The model under review builds one solid part; all positions refer to its coordinate system, in mm. A direction names the side the tool comes from. Give positions to 0.01 mm unless a question says otherwise; leave off trailing zeros. Order: outer loops, then holes, each group sorted by start corner. A loop starts at its lowest first (then second) coordinate and runs counter-clockwise, first axis right, second up. Notation, with made-up numbers: (30, 53.25) - (67, 53.25) arc R8 ccw to (67, 66.25) - close; hole circle Ø5 at (-4.5, 22). An arc over 180 degrees is marked (long way). Write item = value, one per line. Start each with the question number.
1. Machinability: for faces 5 (the cylindrical face through (2.93, 2.12, 10.96)), 6 (the flat face through (-7, -6.9, 6)), 7 (the cylindrical face through (-0.709, 5.828, 3.636)), 8 (the flat face through (16.675, -2, 6)), which of the approach directions +Z, -Z, +X, -X, +Y, -Y give a long, thin tool a straight path to every point of the face, cutting with its end or side? Answer none if there is none.
2. We need section C-C, the plane z = 2.25. Give the boundary of the cut face in (x, y) (3 decimals), and give its area (3 significant figures).
3. We need section B-B, the plane x = -8.5. Give the boundary of the cut face in (y, z).
4. Wall thickness on probe 1 along Y at (x, z) = (-5, 4); probe 2 along X at (y, z) = (-15, 3.5) (3 decimals); probe 3 along Y at (x, z) = (12.5, 1): over which ranges is each line inside the solid? List them lowest first.
5. We need section D-D, the plane x = 7. Give the boundary of the cut face in (y, z), and give its area (3 significant figures).
6. Mouldability with a two-part tool opening along X and no side actions: class faces 1 (the cylindrical face through (-7.226, -5.632, 5.994)), 2 (the flat face through (-10.925, -6, 9)), 3 (the flat face through (5, -12, 0)), 4 (the cylindrical face through (17.776, -5.632, 5.994)) as pulls with the +X half, pulls with the -X half, needs draft (parallel to the pull), parting line crosses it, or undercut.
7. We need section A-A, the plane y = 1. Give the boundary of the cut face in (x, z) (3 decimals), and give its area (3 significant figures).
8. For P1, Ø5, axis at x = 17.5, z = 10.5, coming from the +Y side; P2, Ø4, axis at x = -9.5, z = 4, coming from the -Y side; P3, Ø4, axis at y = -17, z = 2, coming from the -X side (3 decimals), all flat-tipped, find the tip position at first contact; note any pin that passes through.
from build123d import *

# Parameters (mm, degrees)
BOSS_EXTRUDE1_DEPTH = 11.85
BOSS_EXTRUDE2_DEPTH = 4.3
SKETCH4_R           = 2.35
BOSS_EXTRUDE3_DEPTH = 31.3
CUT_EXTRUDE1_DEPTH  = 32.1


with BuildPart() as part:
    # Sketch1 → Boss-Extrude1 (new body)
    with BuildSketch(Plane.XY):
        Polygon((0, 0), (-6.125, 0), (-6.125, -4.4), (-10.925, -4.4), (-10.925, -6.9), (-6.125, -6.9), (-6.125, -23.9), (16.675, -23.9), (16.675, -6.9), (21.175, -6.9), (21.175, -4.4), (16.675, -4.4), (16.675, 0), align=None)
    extrude(amount=BOSS_EXTRUDE1_DEPTH)

    # Boss-Extrude2: read off the stored shape, not the designer's step
    # Boss-Extrude2 outline → Boss-Extrude2 (add)
    with BuildSketch(Plane(origin=(0, 0, 0), x_dir=(1, 0, 0), z_dir=(0, 1, 0))):
        with BuildLine():
            Line((5.048154438, -8.68), (5.62, -8.68))
            ThreePointArc((5.62, -8.68), (8.37, -5.93), (5.62, -3.18))
            Line((5.62, -3.18), (5.048154438, -3.18))
            ThreePointArc((5.048154438, -3.18), (-5.20541828, -2.759603678), (-0.44336187, -11.85))
            Line((-0.44336187, -11.85), (0.04336187, -11.85))
            ThreePointArc((0.04336187, -11.85), (2.970396322, -10.93541828), (5.048154438, -8.68))
        make_face()
    extrude(amount=BOSS_EXTRUDE2_DEPTH)

    # Sketch4 → Boss-Extrude3 (add)
    with BuildSketch(Plane.XZ.offset(23.9)):
        with Locations((-0.2, 5.93)):
            Circle(SKETCH4_R)
    extrude(amount=-BOSS_EXTRUDE3_DEPTH)

    # Sketch5 → Cut-Extrude1 (cut)
    with BuildSketch(Plane(origin=(0, -4.4, 0), x_dir=(1, 0, 0), z_dir=(0, 1, 0))):
        with BuildLine():
            Line((-10.137435839, -5.425), (-10.925, -5.425))
            Line((-10.925, -5.425), (-10.925, -5.925))
            Line((-10.925, -5.925), (-10.925, -6.425))
            Line((-10.925, -6.425), (-10.140971398, -6.425))
            ThreePointArc((-10.140971398, -6.425), (-7.225009375, -5.935303305), (-10.137435839, -5.425))
        make_face()
        with BuildLine():
            Line((20.687435839, -5.425), (21.475, -5.425))
            Line((21.475, -5.425), (21.475, -5.925))
            Line((21.475, -5.925), (21.475, -6.425))
            Line((21.475, -6.425), (20.690971398, -6.425))
            ThreePointArc((20.690971398, -6.425), (17.775009375, -5.935303305), (20.687435839, -5.425))
        make_face()
    extrude(amount=-CUT_EXTRUDE1_DEPTH, mode=Mode.SUBTRACT)


solid = part.part
Model answer:
q1.face_5 = +Z, +X, +Y
q1.face_6 = +Z, -Z, -X, -Y
q1.face_7 = +Y
q1.face_8 = +Z, -Z, +X, +Y
q2.outline = (-10.925, -6.9) - (-6.125, -6.9) - (-6.125, -23.9) - (16.675, -23.9) - (16.675, -6.9) - (21.175, -6.9) - (21.175, -4.4) - (16.675, -4.4) - (16.675, 0) - (4.444, 0) - (4.444, 4.3) - (-4.844, 4.3) - (-4.844, 0) - (-6.125, 0) - (-6.125, -4.4) - (-10.925, -4.4) - close
q2.area = 608 mm2
q3.outline = (-6.9, 0) - (-4.4, 0) - (-4.4, 4.45) - (-6.9, 4.45) - close; (-6.9, 7.41) - (-4.4, 7.41) - (-4.4, 11.85) - (-6.9, 11.85) - close
q4.probe_1 = -23.9 to 4.3
q4.probe_2 = -6.125 to 16.675
q4.probe_3 = -23.9 to 0
q5.outline = (-23.9, 0) - (0, 0) - (0, 3.55) - (4.3, 3.55) - (4.3, 8.31) - (0, 8.31) - (0, 11.85) - (-23.9, 11.85) - close
q5.area = 304 mm2
q6.face_1 = undercut
q6.face_2 = pulls with the -X half
q6.face_3 = needs draft
q6.face_4 = undercut
q7.outline = (-0.443, 11.85) arc R5.925 ccw (long way) to (5.048, 3.18) - (5.62, 3.18) arc R2.75 ccw to (5.62, 8.68) - (5.048, 8.68) arc R5.925 ccw to (0.043, 11.85) - close
q7.area = 123 mm2
q8.P1 = 0
q8.P2 = -6.9
q8.P3 = -6.125
